Verification items for the finished model (mm, model axes). A direction names the side the tool comes from. Give positions to 0.01 mm unless a question says otherwise; leave off trailing zeros. Loops run counter-clockwise (first coordinate to the right, second up) from the corner with the lowest first, then second, coordinate; pieces in that order, holes last. Notation, with made-up numbers: (57.5, -8.5) -> (116.5, -8.5) arc R37 ccw to (116.5, 30.5) -> close; hole circle Ø9 at (64.25, -11.5). An arc over 180 degrees is marked (long way). Use one line per item in the form item = value. Start each with the question number.
Autodesk Inventor part; units mm, degrees
ref_plane "YZ Plane" through (0, 0, 0) normal (1, 0, 0) x (0, 1, 0)
ref_plane "XZ Plane" through (0, 0, 0) normal (0, 1, 0) x (-1, 0, 0)
ref_plane "XY Plane" through (0, 0, 0) normal (0, 0, 1) x (1, 0, 0)
sketch "Sketch1" plane through (0, 0, 0) normal (0, 0, 1) x (1, 0, 0)
  line L0 (-24.5, -12.75) -> (24.5, -12.75)
  line L1 (24.5, -12.75) -> (24.5, 12.75)
  line L2 (24.5, 12.75) -> (-24.5, 12.75)
  line L3 (-24.5, 12.75) -> (-24.5, -12.75)
  line L4 (-24.5, -12.75) -> (24.5, 12.75) construction
  line L5 (24.5, -12.75) -> (-24.5, 12.75) construction
  point P0 (0, 0)
  dimension "d0" = 49
  dimension "d1" = 25.5
extrude "Extrusion1" add sketch "Sketch1" along normal blind 1.6
sketch "Sketch2" plane through (0, 0, 1.6) normal (0, 0, 1) x (1, 0, 0)
  line L0 (-12.5, -9.75) -> (12.5, -9.75)
  line L1 (12.5, -9.75) -> (12.5, 9.75)
  line L2 (12.5, 9.75) -> (-12.5, 9.75)
  line L3 (-12.5, 9.75) -> (-12.5, -9.75)
  line L4 (-12.5, -9.75) -> (12.5, 9.75) construction
  line L5 (12.5, -9.75) -> (-12.5, 9.75) construction
  point P0 (0, 0)
  dimension "d4" = 25
  dimension "d5" = 19.5
extrude "Extrusion2" add sketch "Sketch2" along normal blind 23
sketch "Sketch3" plane through (0, 0, 1.6) normal (0, 0, 1) x (1, 0, 0)
  line L0 (16.75, 2.5) -> (23.25, 2.5)
  line L1 (23.25, 2.5) -> (23.25, -2.5)
  line L2 (23.25, -2.5) -> (16.75, -2.5)
  line L3 (16.75, -2.5) -> (16.75, 2.5)
  line L4 (-23.25, 10) -> (-16.75, 10)
  line L5 (-16.75, 10) -> (-16.75, 5)
  line L6 (-16.75, 5) -> (-23.25, 5)
  line L7 (-23.25, 5) -> (-23.25, 10)
  line L8 (-23.25, -5) -> (-16.75, -5)
  line L9 (-16.75, -5) -> (-16.75, -10)
  line L10 (-16.75, -10) -> (-23.25, -10)
  line L11 (-23.25, -10) -> (-23.25, -5)
  line L12 (24.5, -12.75) -> (24.5, 12.75) construction
  line L13 (-16.75, 5) -> (-16.75, -5) construction
  point P0 (0, 0)
  point P1 (23.25, 0)
  point P2 (-16.75, 0)
  dimension "d8" = 5
  dimension "d9" = 5
  dimension "d10" = 5
  dimension "d11" = 6.5
  dimension "d12" = 6.5
  dimension "d13" = 6.5
  dimension "d14" = 33.5
  dimension "d15" = 1.25
  dimension "d16" = 10
extrude "Extrusion3" add sketch "Sketch3" along normal blind 10
sketch "Sketch4" plane through (0, 0, 1.6) normal (0, 0, 1) x (1, 0, 0)
  line L0 (20, 8.25) -> (20, -8.25) construction
  line L1 (-24.5, 12.75) -> (-24.5, -12.75)
  point P0 (0, 0)
  point P1 (-20, 0)
  point P2 (20, 0)
  dimension "d19" = 40
  dimension "d20" = 16.5
  dimension "d21" = 4.5
hole "Hole1" at (-20, 0, 1.6) at (20, 8.25, 1.6) at (20, -8.25, 1.6) direction (0, 0, -1) diameter 3.4 depth 8 tip angle 118
properties part number "GDT"
Item 1: Sectioned sample at A-A, the plane x = 20. Enter the section's corners in (y, z).
Item 2: Draft check along Y on faces 6 (the flat face through (-20, 5, 7)), 7 (the flat face through (0, -12.75, 1)), 8 (the flat face through (0, 0, 0)). Enter one of: +Y half, -Y half, draft (parallel to the pull), parting line (faces both ways), or undercut.
Item 3: Tool access check on faces 1 (the flat face through (-20, -7, 11.6)), 2 (the flat face through (20, 2.5, 7)), 3 (the flat face through (0, -9.75, 13)), 4 (the flat face through (-16.75, -7, 7)), 5 (the flat face through (-20, -10, 7)). Record the directions out of +Z, -Z, +X, -X, +Y, -Y that give a thin tool (end or side, any length) a straight path to the whole face; none if there is none.
Item 4: Gauge pin test, flat ends, axial feed: pin 1 Ø1.5 at (x, z) = (4, 19.5) entering from +Y; pin 2 Ø2.5 at (x, y) = (-20, 7.5) entering from +Z; pin 3 Ø1 at (y, z) = (-4, 18) entering from +X. Record the tip position at first contact, or that the pin passes through.
Item 5: Material ranges on line 1 (Y direction, x = 20, z = 0.95); line 2 (X direction, y = 0, z = 1.25); line 3 (X direction, y = -8.25, z = 1), recorded low to high.
Item 6: Sectioned sample at C-C, the plane z = 5.5. Enter the section's corners in (x, y).
Item 7: Sectioned sample at D-D, the plane x = 4.5. Enter the section's corners in (y, z), and give its area (3 significant figures).
Item 8: Sectioned sample at B-B, the plane y = 0. Enter the section's corners in (x, z), and give its area (3 significant figures).
Outcome:
q1.outline = (-12.75, 0) -> (-9.95, 0) -> (-9.95, 1.6) -> (-12.75, 1.6) -> close; (-6.55, 0) -> (6.55, 0) -> (6.55, 1.6) -> (2.5, 1.6) -> (2.5, 11.6) -> (-2.5, 11.6) -> (-2.5, 1.6) -> (-6.55, 1.6) -> close; (9.95, 0) -> (12.75, 0) -> (12.75, 1.6) -> (9.95, 1.6) -> close
q2.face_6 = undercut
q2.face_7 = -Y half
q2.face_8 = draft
q3.face_1 = +Z, -X, +Y, -Y
q3.face_2 = +Z, +X, +Y
q3.face_3 = +Z, +X, -Y
q3.face_4 = +Z, +Y, -Y
q3.face_5 = +Z, +X, -X, -Y
q4.pin_1 = 9.75
q4.pin_2 = 11.6
q4.pin_3 = 12.5
q5.line_1 = -12.75 to -9.95, -6.55 to 6.55, 9.95 to 12.75
q5.line_2 = -24.5 to -21.7, -18.3 to 24.5
q5.line_3 = -24.5 to 18.3, 21.7 to 24.5
q6.outline = (-23.25, -10) -> (-16.75, -10) -> (-16.75, -5) -> (-23.25, -5) -> close; (-23.25, 5) -> (-16.75, 5) -> (-16.75, 10) -> (-23.25, 10) -> close; (-12.5, -9.75) -> (12.5, -9.75) -> (12.5, 9.75) -> (-12.5, 9.75) -> close; (16.75, -2.5) -> (23.25, -2.5) -> (23.25, 2.5) -> (16.75, 2.5) -> close
q7.outline = (-12.75, 0) -> (12.75, 0) -> (12.75, 1.6) -> (9.75, 1.6) -> (9.75, 24.6) -> (-9.75, 24.6) -> (-9.75, 1.6) -> (-12.75, 1.6) -> close
q7.area = 489 mm^2
q8.outline = (-24.5, 0) -> (-21.7, 0) -> (-21.7, 1.6) -> (-24.5, 1.6) -> close; (-18.3, 0) -> (24.5, 0) -> (24.5, 1.6) -> (23.25, 1.6) -> (23.25, 11.6) -> (16.75, 11.6) -> (16.75, 1.6) -> (12.5, 1.6) -> (12.5, 24.6) -> (-12.5, 24.6) -> (-12.5, 1.6) -> (-18.3, 1.6) -> close
q8.area = 713 mm^2
